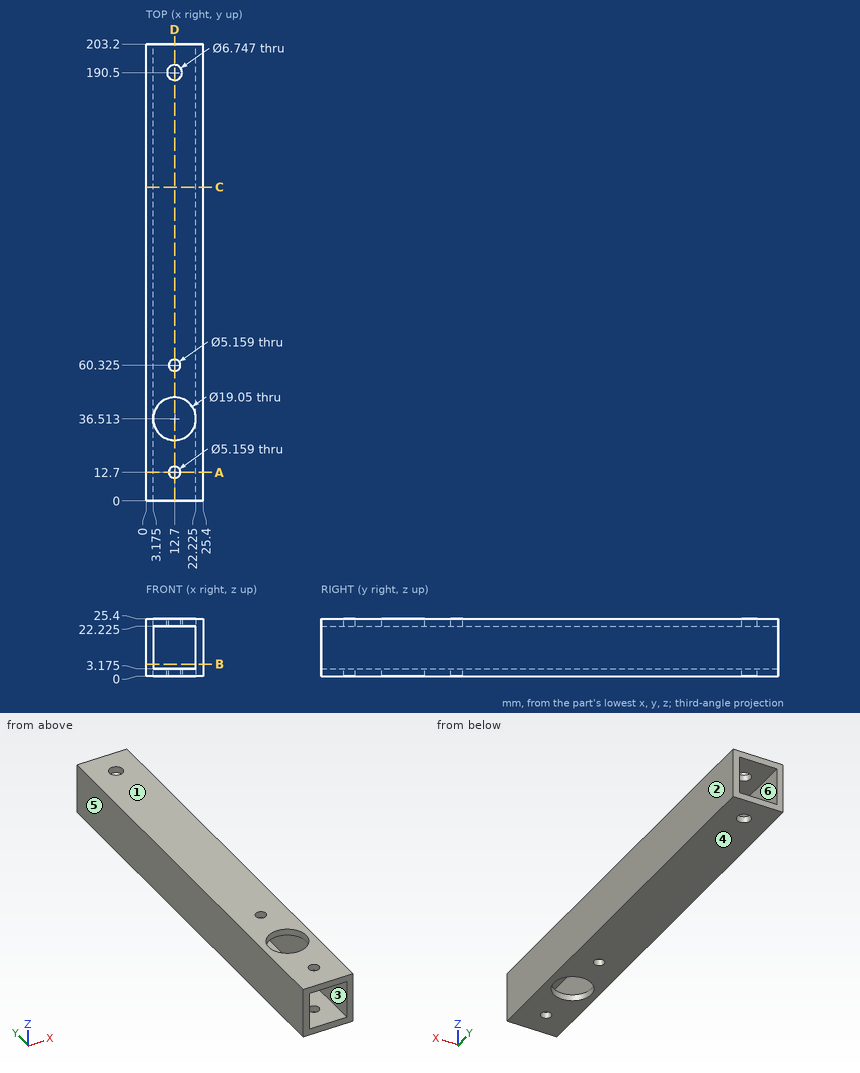
The figure shows three views and two pictorial views of one solid part (mm, origin at its lowest corner). Answer the questions. A direction names the side the tool comes from. Round coordinates to 2 decimals unless told otherwise and drop trailing zeros. Loops run counter-clockwise (first coordinate to the right, second up) from the corner with the lowest first, then second, coordinate; pieces in that order, holes last. Notation, with made-up numbers: (43, 1) - (92, 1) arc R15 ccw to (92, 21) - close; hole circle Ø8 at (55.5, -6.75). An arc over 180 degrees is marked (long way). Use one line per item in the form item = value. Start each with the question number.
(1) Find section A-A on y = 12.7. Determine the outline of the cut face in (x, z) (1 decimal).
(2) Consider line 1 (Y direction, x = 12.7, z = 2.1) (1 decimal); line 2 (X direction, y = 36.5, z = 19.75) (1 decimal). Determine where each line is inside the solid, lowest interval first.
(3) A flat-ended cylindrical pin translates along its axis: P1, Ø4, axis at x = 12.7, y = 12.7, coming from the +Z side. Find the tip coordinate at first contact, or state that the pin passes through.
(4) Find section C-C on y = 139.5. Determine the outline of the cut face in (x, z) (1 decimal).
(5) Determine the mould class of the marked faces 1, 2, 3 and 4 for opening direction Z: +Z half, -Z half, draft (parallel to the pull), parting line (faces both ways), or undercut.
(6) Find section B-B on z = 5.25. Determine the outline of the cut face in (x, y) (1 decimal).
(7) Which of the six approach directions +Z, -Z, +X, -X, +Y, -Y give full straight-line access (tool end or side, diameter ignored) to the marked faces 5 and 6?
(8) Find section D-D on x = 12.7. Give the number of separate pieces and of enclosed holes in the cut face, and give its area (3 significant figures).
Answer list:
q1.outline = (0, 0) - (10.1, 0) - (10.1, 3.2) - (3.2, 3.2) - (3.2, 22.2) - (10.1, 22.2) - (10.1, 25.4) - (0, 25.4) - close; (15.3, 0) - (25.4, 0) - (25.4, 25.4) - (15.3, 25.4) - (15.3, 22.2) - (22.2, 22.2) - (22.2, 3.2) - (15.3, 3.2) - close
q2.line_1 = 0 to 10.1, 15.3 to 27, 46 to 57.7, 62.9 to 187.1, 193.9 to 203.2
q2.line_2 = 0 to 3.2, 22.2 to 25.4
q3.P1 = through
q4.outline = (0, 0) - (25.4, 0) - (25.4, 25.4) - (0, 25.4) - close; hole (3.2, 3.2) - (22.2, 3.2) - (22.2, 22.2) - (3.2, 22.2) - close
q5.face_1 = +Z half
q5.face_2 = draft
q5.face_3 = undercut
q5.face_4 = -Z half
q6.outline = (0, 0) - (3.2, 0) - (3.2, 203.2) - (0, 203.2) - close; (22.2, 0) - (25.4, 0) - (25.4, 203.2) - (22.2, 203.2) - close
q7.face_5 = +Z, -Z, -X, +Y, -Y
q7.face_6 = +Y, -Y
q8.separate_pieces = 10
q8.enclosed_holes = 0
q8.area = 1,060 mm^2
